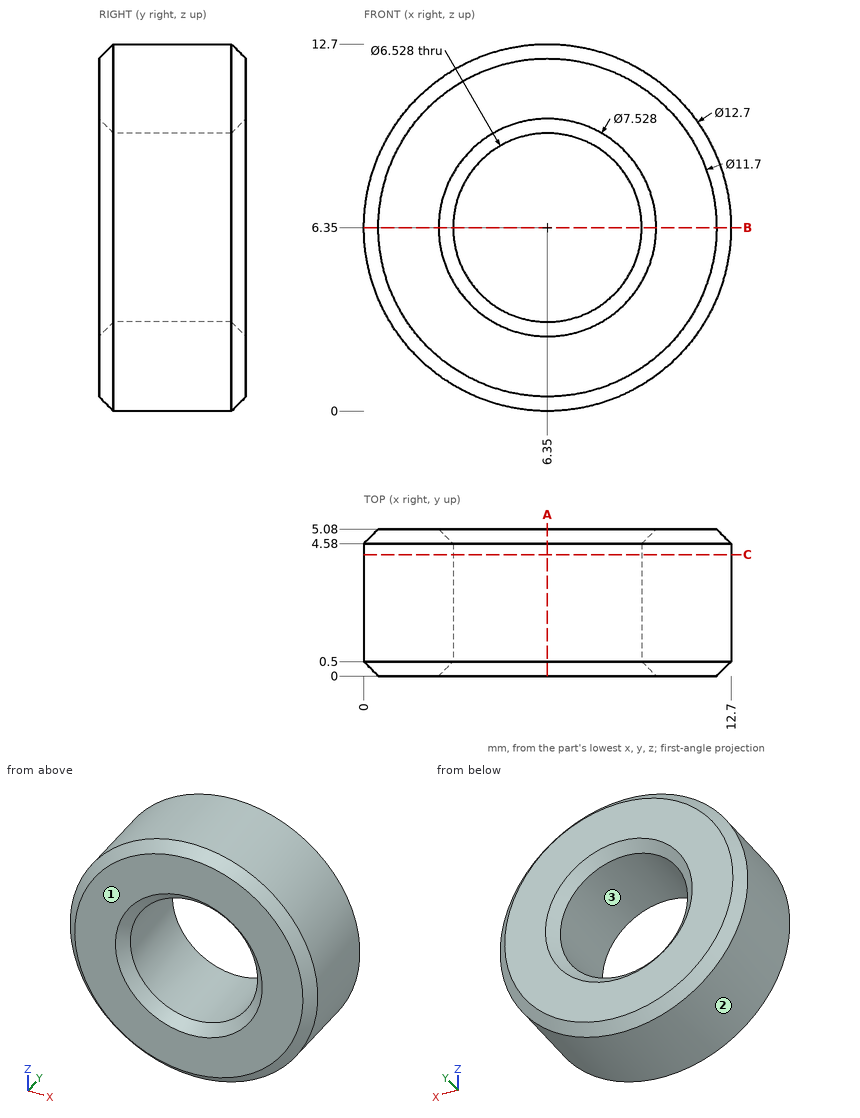
Drawing for the job (mm, zero at the part's lowest x, y, z). Round coordinates to 2 decimals unless told otherwise and drop trailing zeros. Write each loop counter-clockwise with the first axis right and the second up, starting at its lowest first coordinate (ties: lowest second). Pieces come first, ordered by that corner, then holes. Notation, with made-up numbers: M 26.25,-19 L 79.25,-19 A29 ccw 79.25,4 Z; hole C -3.5,80 d6. An arc over 180 degrees is marked long. Put each result on its own line as item: value.
Item 1: Mould opens along Z. For the marked faces 1, 2 and 3 say: +Z half, -Z half, draft (parallel to the pull), parting line (faces both ways), or undercut.
Responses:
face 1: draft
face 2: parting line
face 3: undercut
Item 2: Cut at A-A (x = 6.35). List the corners of the cut face in (y, z).
Responses:
outline: M 0,0.5 L 0.5,0 L 4.58,0 L 5.08,0.5 L 5.08,2.59 L 4.58,3.09 L 0.5,3.09 L 0,2.59 Z; M 0,10.11 L 0.5,9.61 L 4.58,9.61 L 5.08,10.11 L 5.08,12.2 L 4.58,12.7 L 0.5,12.7 L 0,12.2 Z
Item 3: Cut at C-C (y = 4.2). List the corners of the cut face in (x, z).
Responses:
outline: C 6.35,6.35 d12.7; hole C 6.35,6.35 d6.53
Item 4: Cut at B-B (z = 6.35). List the corners of the cut face in (x, y).
Responses:
outline: M 0,0.5 L 0.5,0 L 2.59,0 L 3.09,0.5 L 3.09,4.58 L 2.59,5.08 L 0.5,5.08 L 0,4.58 Z; M 9.61,0.5 L 10.11,0 L 12.2,0 L 12.7,0.5 L 12.7,4.58 L 12.2,5.08 L 10.11,5.08 L 9.61,4.58 Z
Item 5: Probe L1, parallel to X at y = 1.55, z = 6.35; L2, parallel to X at y = 1.35, z = 8.75; L3, parallel to Z at x = 5, y = 1.9 (1 decimal). List the from-to ranges inside material, lowest first. Write a range as from..to.
Responses:
L1: 0..3.09, 9.61..12.7
L2: 0.47..4.14, 8.56..12.23
L3: 0.1..3.4, 9.3..12.6
Item 6: Flat gauge pins, fed straight in: P1, Ø1, axis at y = 2.5, z = 8, coming from the +X side (3 decimals); P2, Ø1, axis at y = 3, z = 10.5, coming from the +X side; P3, Ø2, axis at y = 4, z = 7, coming from the +X side; P4, Ø2, axis at y = 2, z = 9.5, coming from the +X side (3 decimals). Where does each tip first touch, or does it go through?
Responses:
P1: x = 12.595
P2: x = 11.55
P3: x = 12.7
P4: x = 12.325
